Here's how the part is built. I have some questions about the finished solid (model axes, mm). A direction names the side the tool comes from. Round coordinates to 2 decimals unless told otherwise and drop trailing zeros. Loops run counter-clockwise (first coordinate to the right, second up) from the corner with the lowest first, then second, coordinate; pieces in that order, holes last. Notation, with made-up numbers: (79, -16.5) - (130, -16.5) arc R20 ccw to (130, 16.5) - close; hole circle Ø11 at (-28.75, 48.25). An arc over 180 degrees is marked (long way). Answer as a JSON object with one key per item and string values. Group by question number.
1) Will this pin go through, and if not, where does the flat tip stop? P1, Ø12, axis at x = -6.5, z = -7.5, coming from the +Y side.
2) I want a section at B-B, the plane y = 2.75. Please give me the cut outline in (x, z).
3) If I drill on line 1 along X through (y, z) = (0.7, 0); line 2 along Z through (x, y) = (-0.05, 0.9); line 3 along X through (y, z) = (3.25, -8.5), over which ranges is the centre line in solid material (lowest first)? Write a range as [from, to].
4) If we mould it in two halves opening along X, with no side actions, what happens to faces 4 (the face through (-25, 1.8, 0.2)), 5 (the face through (22.5, 5, 8)), 6 (the face through (0, 1, -12.5))? For each: pulls with the +X half, pulls with the -X half, needs draft (parallel to the pull), parting line crosses it, or undercut.
5) Which directions (+Z, -Z, +X, -X, +Y, -Y) give clear straight access to the entire face, cutting with the end or side of a thin tool? Please do faces 1 (the face through (25, 1.8, 0.2)), 2 (the face through (-22.6, 5, -8)), 3 (the face through (-24, 6, -4)).
6) I want a section at C-C, the plane z = -5.75. Please give me the cut outline in (x, y).
7) I want a section at D-D, the plane y = 9. Please give me the cut outline in (x, z), then the cut area to 3 significant figures.
8) I want a section at A-A, the plane x = -0.05. Please give me the cut outline in (y, z).
from build123d import *

# Parameters (mm, degrees)
SKETCH1_W           = 50
SKETCH1_H           = 25
BOSS_EXTRUDE1_DEPTH = 2
SKETCH2_W           = 2.4
SKETCH2_H           = 25
BOSS_EXTRUDE2_DEPTH = 9
CUT_EXTRUDE1_DEPTH  = 9
SKETCH4_W           = 2.5
SKETCH4_H           = 25
BOSS_EXTRUDE3_DEPTH = 9
CUT_EXTRUDE2_DEPTH  = 9
SKETCH6_R           = 2.5
CUT_EXTRUDE4_DEPTH  = 3


with BuildPart() as part:
    # Sketch1 → Boss-Extrude1 (new body)
    with BuildSketch(Plane(origin=(0, 0, 0), x_dir=(1, 0, 0), z_dir=(0, 1, 0))):
        Rectangle(SKETCH1_W, SKETCH1_H)
    extrude(amount=BOSS_EXTRUDE1_DEPTH)

    # Sketch2 → Boss-Extrude2 (add)
    with BuildSketch(Plane(origin=(0, 2, 0), x_dir=(1, 0, 0), z_dir=(0, 1, 0))):
        with Locations((-23.8, 0)):
            Rectangle(SKETCH2_W, SKETCH2_H)
    extrude(amount=BOSS_EXTRUDE2_DEPTH)

    # Sketch3 → Cut-Extrude1 (cut)
    with BuildSketch(Plane(origin=(-22.6, 0, 0), x_dir=(0, 0, -1), z_dir=(1, 0, 0))):
        Polygon((-9, 11), (0, 2), (9, 11), align=None)
    extrude(amount=-CUT_EXTRUDE1_DEPTH, mode=Mode.SUBTRACT)

    # Sketch4 → Boss-Extrude3 (add)
    with BuildSketch(Plane(origin=(0, 2, 0), x_dir=(1, 0, 0), z_dir=(0, 1, 0))):
        with Locations((23.75, 0)):
            Rectangle(SKETCH4_W, SKETCH4_H)
    extrude(amount=BOSS_EXTRUDE3_DEPTH)

    # Sketch5 → Cut-Extrude2 (cut)
    with BuildSketch(Plane.ZY.offset(-22.5)):
        Polygon((0, 2), (-9, 11), (9, 11), align=None)
    extrude(amount=-CUT_EXTRUDE2_DEPTH, mode=Mode.SUBTRACT)

    # Sketch6 → Cut-Extrude4 (cut, through all)
    with BuildSketch(Plane(origin=(0, 2, 0), x_dir=(1, 0, 0), z_dir=(0, 1, 0))):
        with Locations((-0.05, 0)):
            Circle(SKETCH6_R)
    extrude(amount=-CUT_EXTRUDE4_DEPTH, mode=Mode.SUBTRACT)


solid = part.part
Outcome:
{
 "1": {"P1": "y = 2"},
 "2": {"outline": "(-25, -12.5) - (-22.6, -12.5) - (-22.6, -0.75) - (-25, -0.75) - close; (-25, 0.75) - (-22.6, 0.75) - (-22.6, 12.5) - (-25, 12.5) - close; (22.5, -12.5) - (25, -12.5) - (25, -0.75) - (22.5, -0.75) - close; (22.5, 0.75) - (25, 0.75) - (25, 12.5) - (22.5, 12.5) - close"},
 "3": {"line 1": "[-25, -2.55], [2.45, 25]", "line 2": "[-12.5, -2.5], [2.5, 12.5]", "line 3": "[-25, -22.6], [22.5, 25]"},
 "4": {"face 4": "pulls with the -X half", "face 5": "undercut", "face 6": "needs draft"},
 "5": {"face 1": "+Z, -Z, +X, +Y, -Y", "face 2": "+Z, -Z, +Y", "face 3": "+X, -X, +Y"},
 "6": {"outline": "(-25, 0) - (25, 0) - (25, 7.75) - (22.5, 7.75) - (22.5, 2) - (-22.6, 2) - (-22.6, 7.75) - (-25, 7.75) - close"},
 "7": {"outline": "(-25, -12.5) - (-22.6, -12.5) - (-22.6, -7) - (-25, -7) - close; (-25, 7) - (-22.6, 7) - (-22.6, 12.5) - (-25, 12.5) - close; (22.5, -12.5) - (25, -12.5) - (25, -7) - (22.5, -7) - close; (22.5, 7) - (25, 7) - (25, 12.5) - (22.5, 12.5) - close", "area": "53.9 mm^2"},
 "8": {"outline": "(0, -12.5) - (2, -12.5) - (2, -2.5) - (0, -2.5) - close; (0, 2.5) - (2, 2.5) - (2, 12.5) - (0, 12.5) - close"}
}
